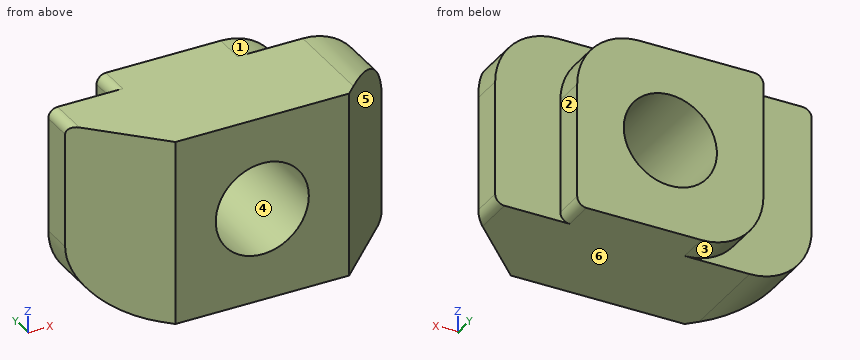
from build123d import *

# Parameters (mm, degrees)
EXTRUDE_1_DEPTH     = 6
FILLET_1_R          = 2
FILLET_2_R          = 2
FILLET_3_R          = 0.3
SKETCH_2_R          = 1.5
CUT_EXTRUDE_1_DEPTH = 6


with BuildPart() as part:
    # 草图1 → 凸台-拉伸1 (new body)
    with BuildSketch(Plane.XY):
        Polygon((-3, 4.3), (3, 4.3), (3, 3.3), (5.1, 3.3), (5.1, 2.3), (2.8, 0), (-2.8, 0), (-5.1, 2.3), (-5.1, 3.3), (-3, 3.3), align=None)
    extrude(amount=EXTRUDE_1_DEPTH)

    # 圆角1
    fillet_1_edges = [part.edges().sort_by_distance(p)[0] for p in [
        (-3, 3.8, 0),
        (3, 3.8, 6),
    ]]
    fillet(fillet_1_edges, radius=FILLET_1_R)

    # 圆角2
    fillet_2_edges = [part.edges().sort_by_distance(p)[0] for p in [
        (-5.1, 2.8, 0),
        (5.1, 2.8, 6),
    ]]
    fillet(fillet_2_edges, radius=FILLET_2_R)

    # 圆角3
    fillet_3_edges = [part.edges().sort_by_distance(p)[0] for p in [
        (-3, 3.8, 6),
        (3, 3.8, 0),
        (-5.1, 2.8, 6),
        (5.1, 2.8, 0),
    ]]
    fillet(fillet_3_edges, radius=FILLET_3_R)

    # 草图2 → 切除-拉伸1 (cut)
    with BuildSketch(Plane(origin=(0, 4.3, 0), x_dir=(1, 0, 0), z_dir=(0, 1, 0))):
        with Locations((0, -3)):
            Circle(SKETCH_2_R)
    extrude(amount=-CUT_EXTRUDE_1_DEPTH, mode=Mode.SUBTRACT)


solid = part.part
Can you work these out from the model? Positions are in its coordinate system, mm. Face numbers are marked on the shaded views. A direction names the side the tool comes from. Round coordinates to 2 decimals unless told otherwise and drop trailing zeros. Order: outer loops, then holes, each group sorted by start corner. A loop starts at its lowest first (then second) coordinate and runs counter-clockwise, first axis right, second up. Notation, with made-up numbers: (-1.75, 55) - (19.25, 55) arc R31 cw to (19.25, 89) - close; hole circle Ø2 at (85.25, -37.75). An arc over 180 degrees is marked (long way). Answer in a Markdown table with one row per item.
(1) Which directions (+Z, -Z, +X, -X, +Y, -Y) give clear straight access to the entire face, cutting with the end or side of a thin tool? Please do the marked faces 1, 2 and 3.
From the geometry:
| item | result |
|---|---|
| face 1 | +Z, +X, +Y |
| face 2 | +Z, -Z, +X, +Y |
| face 3 | -Z, -X, +Y |
(2) Suppose I cut it at A-A, the plane x = 0. Please give me the cut outline in (y, z), plus the area to 3 significant figures.
From the geometry:
| item | result |
|---|---|
| outline | (0, 0) - (4.3, 0) - (4.3, 1.5) - (0, 1.5) - close; (0, 4.5) - (4.3, 4.5) - (4.3, 6) - (0, 6) - close |
| area | 12.9 mm2 |
(3) Suppose I cut it at B-B, the plane z = 3. Please give me the cut outline in (x, y).
From the geometry:
| item | result |
|---|---|
| outline | (-5.1, 2.3) - (-2.8, 0) - (-1.5, 0) - (-1.5, 4.3) - (-3, 4.3) - (-3, 3.3) - (-5.1, 3.3) - close; (1.5, 0) - (2.8, 0) - (5.1, 2.3) - (5.1, 3.3) - (3, 3.3) - (3, 4.3) - (1.5, 4.3) - close |
(4) Please list where these lines run through material, in increasing order: L1, parallel to Z at x = 0, y = 1.8; L2, parallel to X at y = 2.95, z = 3; L3, parallel to X at y = 1, z = 3.75. Write a range as from..to.
From the geometry:
| item | result |
|---|---|
| L1 | z = 0..1.5, 4.5..6 |
| L2 | x = -5.1..-1.5, 1.5..5.1 |
| L3 | x = -3.8..-1.3, 1.3..3.8 |
(5) Suppose I cut it at D-D, the plane z = 1.65. Please give me the cut outline in (x, y), plus the area to 3 significant figures.
From the geometry:
| item | result |
|---|---|
| outline | (-5.07, 2.27) - (-2.8, 0) - (-0.65, 0) - (-0.65, 4.3) - (-2.97, 4.3) - (-2.97, 3.3) - (-5.07, 3.3) - close; (0.65, 0) - (2.8, 0) - (5.1, 2.3) - (5.1, 3.3) - (3, 3.3) - (3, 4.3) - (0.65, 4.3) - close |
| area | 28.7 mm2 |
(6) Suppose I cut it at C-C, the plane y = 1.65. Please give me the cut outline in (x, z).
From the geometry:
| item | result |
|---|---|
| outline | (-4.45, 0.52) arc R2 ccw to (-3.1, 0) - (4.45, 0) - (4.45, 5.48) arc R2 ccw to (3.1, 6) - (-4.45, 6) - close; hole circle Ø3 at (0, 3) |
(7) If we mould it in two halves opening along Z, with no side actions, what happens to the marked faces 4, 5 and 6? For each: released by +Z, released by -Z, zero draft, split by the parting line, or undercut.
From the geometry:
| item | result |
|---|---|
| face 4 | undercut |
| face 5 | zero draft |
| face 6 | released by -Z |
